```python
from build123d import *

# Parameters (mm, degrees)
BOSS_EXTRUDE3_DEPTH  = 3
BOSS_EXTRUDE4_DEPTH  = 150
BOSS_EXTRUDE7_DEPTH  = 150
BOSS_EXTRUDE11_DEPTH = 7.5
SKETCH10_W           = 60
SKETCH10_H           = 50
BOSS_EXTRUDE12_DEPTH = 5
CUT_EXTRUDE1_DEPTH   = 195.89610275
SKETCH12_R           = 1.5
CUT_EXTRUDE2_DEPTH   = 190.831504348


with BuildPart() as part:
    # Sketch2 → Boss-Extrude3 (new body)
    with BuildSketch(Plane(origin=(0, 0, 0), x_dir=(0, 0, -1), z_dir=(1, 0, 0))):
        with BuildLine():
            Line((-2.455878577, 0), (-28, 0))
            ThreePointArc((-28, 0), (-29.414213562, 0.585786438), (-30, 2))
            Line((-30, 2), (-30, 37.959376251))
            ThreePointArc((-30, 37.959376251), (-29.415933658, 39.371867622), (-28.004868125, 39.959370326))
            add(Edge.make_bspline(
                [(-19.566381264, 57.529565551), (-18.600890686, 53.540054818), (-14.629736922, 44.732493893), (-20.209073936, 39.978345831), (-28.004868125, 39.959370326)],
                knots=[0.096883264, 0.096883264, 0.096883264, 0.096883264, 0.548441632, 0.966186264, 0.966186264, 0.966186264, 0.966186264], degree=3))
            ThreePointArc((-19.566381264, 57.529565551), (-19.194257187, 59.23675606), (-17.622495612, 60))
            Line((-17.622495612, 60), (8, 60))
            ThreePointArc((8, 60), (9.414213562, 59.414213562), (10, 58))
            Line((10, 58), (10, 40.744458909))
            ThreePointArc((10, 40.744458909), (9.87713793, 40.054275462), (9.523646809, 39.448889381))
            ThreePointArc((9.523646809, 39.448889381), (0.359945302, 22.023181527), (-0.487300765, 2.353130851))
            ThreePointArc((-0.487300765, 2.353130851), (-0.921886774, 0.716696003), (-2.455878577, 0))
        make_face()
    boss_extrude3 = extrude(amount=BOSS_EXTRUDE3_DEPTH)

    # Sketch3 → Boss-Extrude4 (add)
    with BuildSketch(Plane.ZY):
        with BuildLine():
            Line((18.228025457, 37.529565551), (15.228025457, 37.529565551))
            ThreePointArc((15.228025457, 37.529565551), (13.544434891, 48.402566635), (16.889669649, 58.8842666))
            Line((16.889669649, 58.8842666), (19.566381264, 57.529565551))
            ThreePointArc((19.566381264, 57.529565551), (16.861238321, 47.665807833), (18.228025457, 37.529565551))
        make_face()
    extrude(amount=BOSS_EXTRUDE4_DEPTH)

    # Sketch6 → Boss-Extrude7 (add)
    with BuildSketch(Plane.ZY):
        with BuildLine():
            ThreePointArc((14.728025457, 37.029565551), (4.752130999, 35.940625674), (-5.265723566, 36.529565551))
            ThreePointArc((-5.265723566, 36.529565551), (-4.976948932, 35.028960586), (-5.271974543, 33.529572064))
            ThreePointArc((-5.271974543, 33.529572064), (4.756163556, 32.65403017), (14.728025457, 34.029565551))
            ThreePointArc((14.728025457, 34.029565551), (14.326101668, 35.529565551), (14.728025457, 37.029565551))
        make_face()
    extrude(amount=BOSS_EXTRUDE7_DEPTH)

    # Mirror2: Boss-Extrude3 across plane
    add(boss_extrude3.mirror(Plane.ZY.offset(75)))

    # Sketch9 → Boss-Extrude11 (add, symmetric)
    with BuildSketch(Plane(origin=(-60, 0, 0), x_dir=(0, 0, -1), z_dir=(1, 0, 0))):
        with BuildLine():
            Line((50, -20.470434449), (80, -20.470434449))
            ThreePointArc((80, -20.470434449), (39.119970751, 1.663921764), (5.271974543, 33.529572064))
            ThreePointArc((5.271974543, 33.529572064), (-4.756163556, 32.65403017), (-14.728025457, 34.029565551))
            ThreePointArc((-14.728025457, 34.029565551), (14.190904343, 2.687943249), (50, -20.470434449))
        make_face()
    boss_extrude11 = extrude(amount=BOSS_EXTRUDE11_DEPTH, both=True)

    # Mirror3: Boss-Extrude11 across plane
    add(boss_extrude11.mirror(Plane.ZY.offset(75)))

    # Sketch10 → Boss-Extrude12 (add)
    with BuildSketch(Plane.XZ.offset(20.470434449)):
        with Locations((-75, -65)):
            Rectangle(SKETCH10_W, SKETCH10_H)
    extrude(amount=BOSS_EXTRUDE12_DEPTH)

    # Sketch11 → Cut-Extrude1 (cut, through all)
    with BuildSketch(Plane(origin=(0, -20.470434449, 0), x_dir=(1, 0, 0), z_dir=(0, 1, 0))):
        with BuildLine():
            Line((-93.7, 87), (-83, 87))
            ThreePointArc((-83, 87), (-81.35, 85.35), (-83, 83.7))
            Line((-83, 83.7), (-93.7, 83.7))
            ThreePointArc((-93.7, 83.7), (-95.35, 85.35), (-93.7, 87))
        make_face()
        with BuildLine():
            Line((-67, 87), (-56.3, 87))
            ThreePointArc((-56.3, 87), (-54.65, 85.35), (-56.3, 83.7))
            Line((-56.3, 83.7), (-67, 83.7))
            ThreePointArc((-67, 83.7), (-68.65, 85.35), (-67, 87))
        make_face()
    extrude(amount=-CUT_EXTRUDE1_DEPTH, mode=Mode.SUBTRACT)

    # Sketch12 → Cut-Extrude2 (cut, through all)
    with BuildSketch(Plane(origin=(3, 0, 0), x_dir=(0, 0, -1), z_dir=(1, 0, 0))):
        with Locations((2, 52)):
            Circle(SKETCH12_R)
        with Locations((-27.5, 15)):
            Circle(SKETCH12_R)
    extrude(amount=-CUT_EXTRUDE2_DEPTH, mode=Mode.SUBTRACT)


solid = part.part
```
Can you work these out from the model? Positions are in its coordinate system, mm. A direction names the side the tool comes from. Give positions to 0.01 mm unless a question says otherwise; leave off trailing zeros. Order: outer loops, then holes, each group sorted by start corner. A loop starts at its lowest first (then second) coordinate and runs counter-clockwise, first axis right, second up. Notation, with made-up numbers: (-1.75, -30.75) - (54.25, -30.75) arc R15 cw to (54.25, -14.75) - close; hole circle Ø5 at (-39.75, -32.5). An arc over 180 degrees is marked (long way). Use a Markdown table: item, result. Add a question column.
Q1. If we section it at A-A on x = -49: Write out the boundary of the cut face in (y, z), plus the area to 3 significant figures.
Q2. I'm going to push flat-ended pins straight in: pin 1 (1.5 mm diameter, centred on x = 1, z = 13, fed in from -Y); pin 2 (1 mm diameter, centred on x = -15, z = -2, fed in from +Y); pin 3 (12 mm diameter, centred on y = 4.5, z = -25, fed in from -X). Where does each tip first touch, or does it pass through?
Q3. If we section it at D-D on z = -69: Write out the boundary of the cut face in (x, y), plus the area to 3 significant figures.
Q4. If we section it at C-C on x = -86.5: Write out the boundary of the cut face in (y, z).
Q5. If we section it at B-B on z = -46: Write out the boundary of the cut face in (x, y).
Q6. On a 3-axis mill with a long thin cutter (end or side, diameter ignored), from which of +Z, -Z, +X, -X, +Y, -Y can I reach the whole of each face in a straight line? I mean faces 4 (the cylindrical face through (-54.65, -22.94, -85.39)), 5 (the cylindrical face through (-25.88, 32.65, 4.61)), 6 (the cylindrical face through (1.479, 22.291, -0.433)). Say none if no direction works.
Q7. If we mould it in two halves opening along X, with no side actions, what happens to faces 1 (the cylindrical face through (-74.9, 32.65, 4.61)), 2 (the flat face through (3, 30, 10)), 3 (the flat face through (-75, -23, -40))? For each: released by +X, released by -X, zero draft, split by the parting line, or undercut.
Q8. Please list where these lines run through material, in increasing order: line 1 along X through (y, z) = (23, 21); line 2 along X through (y, z) = (-10, -43); line 3 along Y through (x, z) = (1.4, 27.5).
Answers follow:
| question | item | result |
|---|---|---|
| 1 | outline | (-25.47, -90) - (-20.47, -90) - (-20.47, -40) - (-25.47, -40) - close; (33.53, -5.27) arc R4 cw to (36.53, -5.27) arc R60 cw to (37.03, 14.73) arc R3 cw to (34.03, 14.73) arc R45 ccw to start; (37.53, 15.23) arc R24 ccw to (58.88, 16.89) - (57.53, 19.57) arc R25.63 cw to (37.53, 18.23) - close |
| 1 | area | 381 mm^2 |
| 2 | pin 1 | stops at y = 0 |
| 2 | pin 2 | stops at y = 36.2 |
| 2 | pin 3 | stops at x = -97.5 |
| 3 | outline | (-105, -25.47) - (-45, -25.47) - (-45, -20.47) - (-52.5, -20.47) - (-52.5, -15.82) - (-67.5, -15.82) - (-67.5, -20.47) - (-82.5, -20.47) - (-82.5, -15.82) - (-97.5, -15.82) - (-97.5, -20.47) - (-105, -20.47) - close |
| 3 | area | 439 mm^2 |
| 4 | outline | (-25.47, -90) - (-20.47, -90) - (-20.47, -87) - (-25.47, -87) - close; (-25.47, -83.7) - (-20.47, -83.7) - (-20.47, -80) arc R180 cw to (33.53, -5.27) arc R4 cw to (36.53, -5.27) arc R60 cw to (37.03, 14.73) arc R3 cw to (34.03, 14.73) arc R170 ccw to (-20.47, -50) - (-20.47, -40) - (-25.47, -40) - close; (37.53, 15.23) arc R24 ccw to (58.88, 16.89) - (57.53, 19.57) arc R25.63 cw to (37.53, 18.23) - close |
| 5 | outline | (-105, -25.47) - (-45, -25.47) - (-45, -20.47) - (-105, -20.47) - close; (-97.5, -18.48) - (-82.5, -18.48) - (-82.5, -3.07) - (-97.5, -3.07) - close; (-67.5, -18.48) - (-52.5, -18.48) - (-52.5, -3.07) - (-67.5, -3.07) - close |
| 6 | face 4 | +Y, -Y |
| 6 | face 5 | -Y |
| 6 | face 6 | -Z, +X |
| 7 | face 1 | undercut |
| 7 | face 2 | released by +X |
| 7 | face 3 | zero draft |
| 8 | line 1 | x = -153 to -150, 0 to 3 |
| 8 | line 2 | x = -97.5 to -82.5, -67.5 to -52.5 |
| 8 | line 3 | y = 0 to 13.5, 16.5 to 39.96 |
